Geometry: final body of the model. Coordinates: model frame, mm. A direction names the side the tool comes from. Round coordinates to 2 decimals unless told otherwise and drop trailing zeros. Write each loop counter-clockwise with the first axis right and the second up, starting at its lowest first coordinate (ties: lowest second). Pieces come first, ordered by that corner, then holes. Notation, with made-up numbers: (35.5, -1.5) - (65.5, -1.5) arc R26 ccw to (65.5, 33.5) - close; hole circle Ø1 at (68, -21). An arc over 180 degrees is marked (long way). Write each question's results on one line, items separated by ' | '.
from build123d import *

# Parameters (mm, degrees)
SKETCH_1_R          = 6.5
EXTRUDE_1_DEPTH     = 5
SKETCH_2_W          = 2.2
SKETCH_2_H          = 2.6
CUT_EXTRUDE_1_DEPTH = 6.95
SKETCH_3_R          = 4
EXTRUDE_2_DEPTH     = 30


with BuildPart() as part:
    # Эскиз1 → Бобышка-Вытянуть1 (new body)
    with BuildSketch(Plane(origin=(0, 0, 0), x_dir=(1, 0, 0), z_dir=(0, 1, 0))):
        with Locations(Location((0, 0, 0), (0, 0, 270))):
            Circle(SKETCH_1_R)
    extrude(amount=EXTRUDE_1_DEPTH)

    # Эскиз2 → Вырез-Вытянуть1 (cut, symmetric)
    with BuildSketch(Plane.XY):
        with Locations((0, 1.3)):
            Rectangle(SKETCH_2_W, SKETCH_2_H)
    extrude(amount=CUT_EXTRUDE_1_DEPTH, both=True, mode=Mode.SUBTRACT)

    # Эскиз3 → Бобышка-Вытянуть2 (add)
    with BuildSketch(Plane(origin=(0, 5, 0), x_dir=(1, 0, 0), z_dir=(0, 1, 0))):
        with Locations(Location((0, 0, 0), (0, 0, 270))):
            Circle(SKETCH_3_R)
    extrude(amount=EXTRUDE_2_DEPTH)


solid = part.part
Q1. Mould query, pull axis X, two halves, no side actions, for faces 3 (the cylindrical face through (-3.905, 19.79, -0.867)), 4 (the flat face through (3, 5, 3)), 5 (the flat face through (0, 2.6, 0)), 6 (the flat face through (1.1, 1, 0)). Classes: pulls with the +X half, pulls with the -X half, needs draft (parallel to the pull), parting line crosses it, or undercut.
Answer block:
face 3: parting line crosses it | face 4: needs draft | face 5: undercut | face 6: undercut
Q2. Ray query, line 1 along Y through (x, z) = (-2.25, 4); line 2 along Z through (x, y) = (-0.25, 15); line 3 along Y through (x, z) = (0, -3.5). Return the intervals inside material, ascending.
Answer block:
line 1: 0 to 5 | line 2: -3.99 to 3.99 | line 3: 2.6 to 35
Q3. Pin query (flat end, axial travel): pin 1 (4 mm diameter, centred on x = 4.5, y = 5, fed in from +Z); pin 2 (5 mm diameter, centred on x = -4.5, y = 26.5, fed in from +Z); pin 3 (3 mm diameter, centred on y = 2, z = 1.5, fed in from +X); pin 4 (0.8 mm diameter, centred on y = 1.5, z = -1.5, fed in from -X). Return the tip coordinate at first contact, or that it passes through.
Answer block:
pin 1: z = 6 | pin 2: z = 3.46 | pin 3: x = 6.5 | pin 4: x = -6.41
Q4. Access query for faces 1 (the cylindrical face through (1.95, 2.46, 6.2)), 2 (the flat face through (-1.1, 1, 0)). Directions: +Z, -Z, +X, -X, +Y, -Y. A direction counts if a zero-diameter tool reaches every point of the face in a straight line with its end or side. Return the directions, or none.
Answer block:
face 1: +Y, -Y | face 2: +Z, -Z, -Y
Q5. Section query A-A, the plane z = 0. Return loops of the section in (x, y), plus the area to 3 significant figures.
Answer block:
outline: (-6.5, 0) - (-1.1, 0) - (-1.1, 2.6) - (1.1, 2.6) - (1.1, 0) - (6.5, 0) - (6.5, 5) - (4, 5) - (4, 35) - (-4, 35) - (-4, 5) - (-6.5, 5) - close | area: 299 mm2
Q6. Section query C-C, the plane y = 28. Return loops of the section in (x, z), plus the area to 3 significant figures.
Answer block:
outline: circle Ø8 at (0, 0) | area: 50.3 mm2
Q7. Section query D-D, the plane x = 2.75. Return loops of the section in (y, z), plus the area to 3 significant figures.
Answer block:
outline: (0, -5.89) - (5, -5.89) - (5, -2.9) - (35, -2.9) - (35, 2.9) - (5, 2.9) - (5, 5.89) - (0, 5.89) - close | area: 233 mm2
Q8. Section query B-B, the plane x = 0. Return loops of the section in (y, z), plus the area to 3 significant figures.
Answer block:
outline: (2.6, -6.5) - (5, -6.5) - (5, -4) - (35, -4) - (35, 4) - (5, 4) - (5, 6.5) - (2.6, 6.5) - close | area: 271 mm2
